from build123d import *

# Parameters (mm, degrees)
EXTRUDE_1_DEPTH = 3
FILLET_1_R      = 5


with BuildPart() as part:
    # 草图1 → 凸台-拉伸1 (new body)
    with BuildSketch(Plane(origin=(0, 0, 0), x_dir=(1, 0, 0), z_dir=(0, 1, 0))):
        Polygon((10, 15), (30, 15), (30, -15), (10, -15), (10, -30), (-10, -30), (-10, -15), (-30, -15), (-30, 15), (-10, 15), (-10, 30), (10, 30), align=None)
    extrude(amount=EXTRUDE_1_DEPTH)

    # 圆角1
    fillet_1_edges = [part.edges().sort_by_distance(p)[0] for p in [
        (10, 1.5, 30),
        (-10, 1.5, 30),
        (-10, 1.5, 15),
        (-30, 1.5, 15),
        (-30, 1.5, -15),
        (-10, 1.5, -15),
        (-10, 1.5, -30),
        (10, 1.5, -30),
        (10, 1.5, -15),
        (30, 1.5, -15),
        (30, 1.5, 15),
        (10, 1.5, 15),
    ]]
    fillet(fillet_1_edges, radius=FILLET_1_R)


solid = part.part
Could you check a few things on this model? Use its own coordinates, in mm. A direction names the side the tool comes from. Give positions to 0.01 mm unless a question says otherwise; leave off trailing zeros. Order: outer loops, then holes, each group sorted by start corner. A loop starts at its lowest first (then second) coordinate and runs counter-clockwise, first axis right, second up. Notation, with made-up numbers: (34.5, 85) - (69.5, 85) arc R15 cw to (69.5, 110) - close; hole circle Ø1 at (29, 9). An arc over 180 degrees is marked (long way). Return JSON: item names as keys, results as strings. Group by question number.
Q1. Suppose I cut it at B-B, the plane z = 13. Please give me the cut outline in (x, y), and give its area (3 significant figures).
Q2. Will these pins go through, and if not, where does the flat tip stop? pin 1 Ø0.9 at (x, y) = (19.5, 1) entering from -Z; pin 2 Ø1.5 at (y, z) = (1.5, 23.5) entering from -X; pin 3 Ø1.5 at (x, z) = (-0.5, -4) entering from -Y; pin 4 Ø1.5 at (y, z) = (1, -23) entering from +X.
Q3. Suppose I cut it at C-C, the plane x = -23. Please give me the cut outline in (y, z).
Q4. Please list where these lines run through material, in increasing order: line 1 along Z through (x, y) = (21.5, 0.65); line 2 along X through (y, z) = (1.8, 23.5); line 3 along Z through (x, y) = (7.5, 1.7). Write a range as [from, to].
Q5. Which directions (+Z, -Z, +X, -X, +Y, -Y) give clear straight access to the entire face, cutting with the end or side of a thin tool? Please do faces 1 (the face through (20, 1, -15)), 2 (the face through (-20, 1, 15)), 3 (the face through (0, 1, 30)), 4 (the face through (10, 1, 22)), 5 (the face through (-20, 1, -15)).
Q6. Suppose I cut it at A-A, the plane y = 0.9. Please give me the cut outline in (x, z), and give its area (3 significant figures).
Resolved:
{
 "1": {"outline": "(-29, 0) - (29, 0) - (29, 3) - (-29, 3) - close", "area": "174 mm2"},
 "2": {"pin 1": "stops at z = -15", "pin 2": "stops at x = -10", "pin 3": "stops at y = 0", "pin 4": "stops at x = 10"},
 "3": {"outline": "(0, -15) - (3, -15) - (3, 15) - (0, 15) - close"},
 "4": {"line 1": "z = [-15, 15]", "line 2": "x = [-10, 10]", "line 3": "z = [-29.33, 29.33]"},
 "5": {"face 1": "-Z, +X, +Y, -Y", "face 2": "+Z, -X, +Y, -Y", "face 3": "+Z, +X, -X, +Y, -Y", "face 4": "+Z, +X, +Y, -Y", "face 5": "-Z, -X, +Y, -Y"},
 "6": {"outline": "(-30, -10) arc R5 ccw to (-25, -15) - (-15, -15) arc R5 cw to (-10, -20) - (-10, -25) arc R5 ccw to (-5, -30) - (5, -30) arc R5 ccw to (10, -25) - (10, -20) arc R5 cw to (15, -15) - (25, -15) arc R5 ccw to (30, -10) - (30, 10) arc R5 ccw to (25, 15) - (15, 15) arc R5 cw to (10, 20) - (10, 25) arc R5 ccw to (5, 30) - (-5, 30) arc R5 ccw to (-10, 25) - (-10, 20) arc R5 cw to (-15, 15) - (-25, 15) arc R5 ccw to (-30, 10) - close", "area": "2,380 mm2"}
}
